Answer from the drawing. Dimensions are ordinates in mm from the lowest x, y and z of the part. Round coordinates to 2 decimals unless told otherwise and drop trailing zeros. Loops run counter-clockwise (first coordinate to the right, second up) from the corner with the lowest first, then second, coordinate; pieces in that order, holes last.
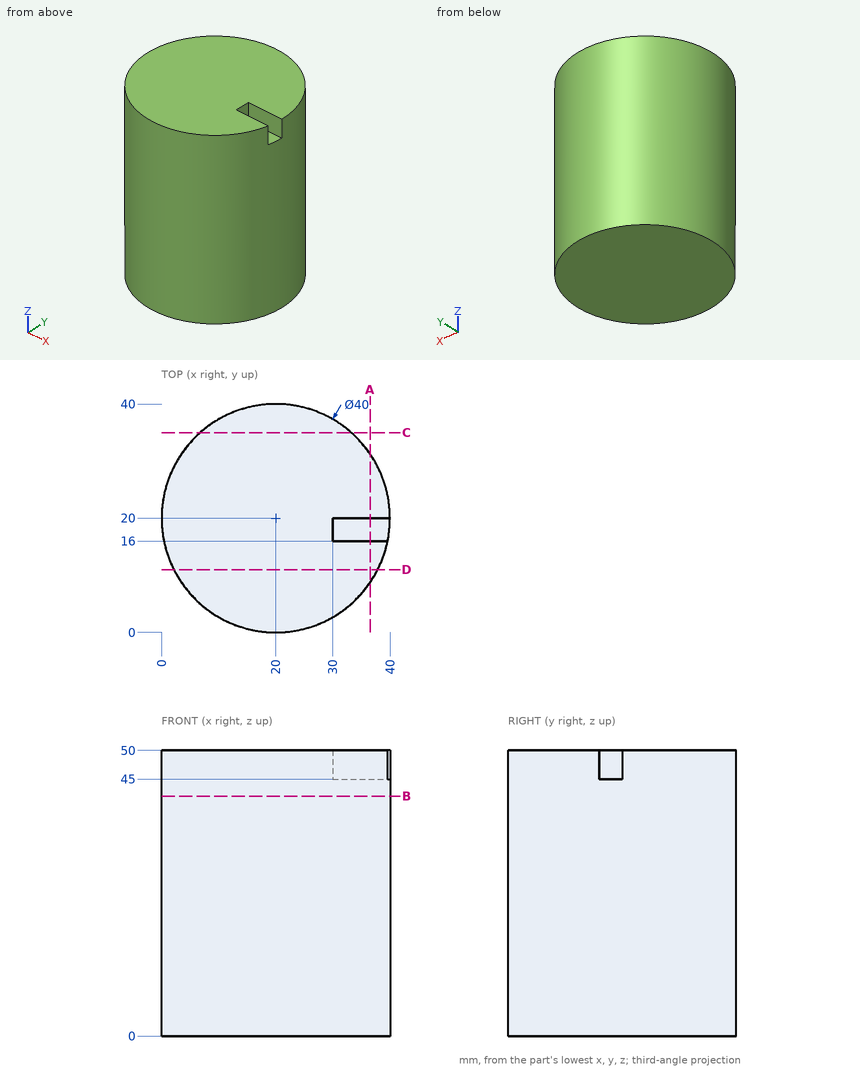
Item 1: Section C-C, the plane y = 35 is taken. Give the vertices of the cut face in (x, z).
Item 2: Section A-A, the plane x = 36.5 is taken. Give the vertices of the cut face in (y, z).
Item 3: Straight lines are drawn through the part: line 1 (X direction, y = 32, z = 15); line 2 (Y direction, x = 31, z = 13.5); line 3 (Y direction, x = 14.5, z = 36). For each, find the intervals that lie inside material, in ascending order.
Item 4: Section B-B, the plane z = 42 is taken. Give the vertices of the cut face in (x, y).
Item 5: Each of these flat-tipped pins is pushed along its axis until it touches: P1, Ø3, axis at x = 29, z = 31.5, coming from the +Y side; P2, Ø5.5, axis at x = 33, z = 46.5, coming from the -Y side; P3, Ø10, axis at x = 32, z = 30, coming from the -Y side (3 decimals). Where does it stop, or does it pass through?
Item 6: Section D-D, the plane y = 11 is taken. Give the vertices of the cut face in (x, z), plus the area to 3 significant figures.
Answer below:
1. outline: (6.77, 0) - (33.23, 0) - (33.23, 50) - (6.77, 50) - close
2. outline: (8.7, 0) - (31.3, 0) - (31.3, 50) - (20, 50) - (20, 45) - (16, 45) - (16, 50) - (8.7, 50) - close
3. line 1: x = 4 to 36
3. line 2: y = 3.3 to 36.7
3. line 3: y = 0.77 to 39.23
4. outline: circle Ø40 at (20, 20)
5. P1: stops at y = 38.54
5. P2: stops at y = 2.83
5. P3: stops at y = 1.265
6. outline: (2.14, 0) - (37.86, 0) - (37.86, 50) - (2.14, 50) - close
6. area: 1,790 mm2
